Input: part model. Units: mm. Frame: model coordinates. A direction names the side the tool comes from. Coordinates: 2 decimals unless noted, no trailing zeros. Loops run counter-clockwise (first coordinate to the right, second up) from the corner with the lowest first, then second, coordinate; pieces in that order, holes last.
(1) Contact query for flat-ended pins moving along their axis: P1, Ø2, axis at x = 1, z = 107.5, coming from the -Y side; P2, Ø8, axis at x = 37.5, z = -21.5, coming from the +Y side; P3, Ø1.6, axis at x = 24, z = -233.5, coming from the -Y side; P4, Ø2, axis at x = 2, y = -2.5, coming from the +Z side. Output: stop coordinate, or through.
(2) Section A-A, the plane z = 152. Return loops of the section in (x, y).
(3) Set-up query: faces 1 (the face through (-35, -28, 3)), 2 (the face through (35, -30, 3)), 3 (the face through (-23.5, -14, 3)). Return all of +Z, -Z, +X, -X, +Y, -Y with unobstructed straight access to the full face (end or side cutting, diameter ignored); none if empty.
(4) Line query: L1, parallel to Z at x = 35.5, y = -29.25; L2, parallel to Z at x = -24, y = -18; L3, parallel to X at y = -29.5, z = -227. Output: solid intervals per line, ascending.
(5) Mould query, pull axis X, two halves, no side actions, for faces 4 (the face through (36, -28, 3)), 5 (the face through (23.5, -14, 3)), 6 (the face through (25.5, -14, 3)), 7 (the face through (-25.5, -14, 3)). Classes: released by +X, released by -X, zero draft, split by the parting line, or undercut.
```python
from build123d import *

# Parameters (mm, degrees)
SM_BASE_FLANGE_1_DEPTH   = 248
SKETCH_7_W               = 35
SKETCH_7_H               = 4
CUT_EXTRUDE_1_DEPTH      = 4
SKETCH_8_W               = 35
SKETCH_8_H               = 4
CUT_EXTRUDE_2_DEPTH      = 4
SKETCH_9_R               = 2.5
CUT_EXTRUDE_3_DEPTH      = 4
SKETCH_11_W              = 8.403654654
SKETCH_11_H              = 30.785672442
SKETCH_11_H_2            = 25.612573904
SM_BASE_FLANGE_1_2_DEPTH = 2
CUT_EXTRUDE_5_DEPTH      = 259.636810992
CUT_EXTRUDE_5_DEPTH_BACK = 259.636810992
SKETCH_14_R              = 3.5


# Sheet-metal steps are written as plain solids
with BuildPart() as part:
    # Sketch 1 → Sm Base Flange 1 (new, symmetric)
    with BuildSketch(Plane.XY):
        with BuildLine():
            Line((-43.5, -30), (-27.5, -30))
            ThreePointArc((-27.5, -30), (-24.671572875, -28.828427125), (-23.5, -26))
            Line((-23.5, -26), (-23.5, -2))
            ThreePointArc((-23.5, -2), (-22.914213562, -0.585786438), (-21.5, 0))
            Line((-21.5, 0), (21.5, 0))
            ThreePointArc((21.5, 0), (22.914213562, -0.585786438), (23.5, -2))
            Line((23.5, -2), (23.5, -26))
            ThreePointArc((23.5, -26), (24.671572875, -28.828427125), (27.5, -30))
            Line((27.5, -30), (43.5, -30))
            Line((43.5, -30), (43.5, -28))
            Line((43.5, -28), (27.5, -28))
            ThreePointArc((27.5, -28), (26.085786438, -27.414213562), (25.5, -26))
            Line((25.5, -26), (25.5, -2))
            ThreePointArc((25.5, -2), (24.328427125, 0.828427125), (21.5, 2))
            Line((21.5, 2), (-21.5, 2))
            ThreePointArc((-21.5, 2), (-24.328427125, 0.828427125), (-25.5, -2))
            Line((-25.5, -2), (-25.5, -26))
            ThreePointArc((-25.5, -26), (-26.085786438, -27.414213562), (-27.5, -28))
            Line((-27.5, -28), (-43.5, -28))
            Line((-43.5, -28), (-43.5, -30))
        make_face()
    extrude(amount=SM_BASE_FLANGE_1_DEPTH, both=True)

    # Эскиз7 → Вырез-Вытянуть1 (cut)
    with BuildSketch(Plane.ZY.offset(-23.5)):
        with Locations((230.5, -28)):
            Rectangle(SKETCH_7_W, SKETCH_7_H)
        with Locations((-230.5, -28)):
            Rectangle(SKETCH_7_W, SKETCH_7_H)
    extrude(amount=-CUT_EXTRUDE_1_DEPTH, mode=Mode.SUBTRACT)

    # Эскиз8 → Вырез-Вытянуть2 (cut)
    with BuildSketch(Plane(origin=(-23.5, 0, 0), x_dir=(0, 0, -1), z_dir=(1, 0, 0))):
        with Locations((230.5, -28)):
            Rectangle(SKETCH_8_W, SKETCH_8_H)
        with Locations((-230.5, -28)):
            Rectangle(SKETCH_8_W, SKETCH_8_H)
    extrude(amount=-CUT_EXTRUDE_2_DEPTH, mode=Mode.SUBTRACT)

    # Эскиз9 → Вырез-Вытянуть3 (cut)
    with BuildSketch(Plane(origin=(0, -28, 0), x_dir=(1, 0, 0), z_dir=(0, 1, 0))):
        with Locations(Location((-35.5, 227, 0), (0, 0, 180))):
            Circle(SKETCH_9_R)
        with Locations(Location((-34.5, 195, 0), (0, 0, 180))):
            Circle(SKETCH_9_R)
        with Locations(Location((-34.5, 179, 0), (0, 0, 180))):
            Circle(SKETCH_9_R)
        with Locations((-34.5, -179)):
            Circle(SKETCH_9_R)
        with Locations((-34.5, -195)):
            Circle(SKETCH_9_R)
        with Locations((-35.5, -227)):
            Circle(SKETCH_9_R)
        with Locations((35.5, 227)):
            Circle(SKETCH_9_R)
        with Locations(Location((35.5, -227, 0), (0, 0, 180))):
            Circle(SKETCH_9_R)
    extrude(amount=-CUT_EXTRUDE_3_DEPTH, mode=Mode.SUBTRACT)

    # Эскиз11 → Sm Base Flange 1 2 (add)
    with BuildSketch(Plane(origin=(0, -28, 0), x_dir=(1, 0, 0), z_dir=(0, 1, 0))):
        with Locations((-34.752058472, -185.409493447)):
            Rectangle(SKETCH_11_W, SKETCH_11_H)
        with Locations((-34.752058472, 186.746789547)):
            Rectangle(SKETCH_11_W, SKETCH_11_H_2)
    extrude(amount=-SM_BASE_FLANGE_1_2_DEPTH)

    # Эскиз14 → Вырез-Вытянуть5 (cut, two sides: drawn at the far end of the back side and taken through both)
    with BuildSketch(Plane(origin=(-23.5, 0, 0), x_dir=(0, 0, -1), z_dir=(1, 0, 0)).offset(-CUT_EXTRUDE_5_DEPTH_BACK)):
        with Locations(Location((-163, -18, 0), (0, 0, 90))):
            Circle(SKETCH_14_R)
        with Locations(Location((-123, -18, 0), (0, 0, 90))):
            Circle(SKETCH_14_R)
        with Locations(Location((123, -18, 0), (0, 0, 90))):
            Circle(SKETCH_14_R)
        with Locations(Location((163, -18, 0), (0, 0, 90))):
            Circle(SKETCH_14_R)
    extrude(amount=CUT_EXTRUDE_5_DEPTH + CUT_EXTRUDE_5_DEPTH_BACK, mode=Mode.SUBTRACT)


solid = part.part
```
Report:
1. P1: stops at y = 0
1. P2: stops at y = -28
1. P3: stops at y = -26
1. P4: passes through
2. outline: (-43.5, -30) - (-27.5, -30) arc R4 ccw to (-23.5, -26) - (-23.5, -2) arc R2 cw to (-21.5, 0) - (21.5, 0) arc R2 cw to (23.5, -2) - (23.5, -26) arc R4 ccw to (27.5, -30) - (43.5, -30) - (43.5, -28) - (27.5, -28) arc R2 cw to (25.5, -26) - (25.5, -2) arc R4 ccw to (21.5, 2) - (-21.5, 2) arc R4 ccw to (-25.5, -2) - (-25.5, -26) arc R2 cw to (-27.5, -28) - (-43.5, -28) - close
3. face 1: +Z, -Z, -X, +Y
3. face 2: +Z, -Z, +X, -X, -Y
3. face 3: +Z, -Z, -Y
4. L1: z = -248 to -229.5, -224.5 to 224.5, 229.5 to 248
4. L2: z = -248 to -166.5, -159.5 to -126.5, -119.5 to 119.5, 126.5 to 159.5, 166.5 to 248
4. L3: x = -43.5 to -38, -33 to -27.5, 27.5 to 33, 38 to 43.5
5. face 4: zero draft
5. face 5: undercut
5. face 6: released by +X
5. face 7: released by -X
